The model under review builds one solid part; all positions refer to its coordinate system, in mm. Face numbers are marked on the shaded views. A direction names the side the tool comes from. Round coordinates to 2 decimals unless told otherwise and drop trailing zeros. Order: outer loops, then holes, each group sorted by start corner. A loop starts at its lowest first (then second) coordinate and runs counter-clockwise, first axis right, second up. Notation, with made-up numbers: M 8,24 L 39,24 A14 cw 39,31 Z; hole C 82.5,66 d7. An arc over 180 degrees is marked long. Use a Markdown table: item, result. Add a question column.
1. Insertion check: P1, Ø6, axis at x = 2.5, z = -22.5, coming from the +Y side; P2, Ø1, axis at x = -2, y = -2, coming from the -Z side; P3, Ø2, axis at x = 1, y = -0.5, coming from the -Z side; P4, Ø5.5, axis at x = 0.5, z = 0, coming from the -Y side. Each pin has a flat end and moves straight along its axis. Give the tip position at first contact, or say it passes through.
2. Consider section C-C on y = 0.75. State the section outline as (x, z) points.
3. Consider section A-A on x = 0. Count the separate pieces of the cut face and the enclosed holes in it, then the cut area to 3 significant figures.
4. Consider section B-B on z = 0. State the section outline as (x, y) points, then the cut area to 3 significant figures.
5. To check wall thickness, follow probe 1 along Z at (x, y) = (0, 0.15); probe 2 along Z at (x, y) = (0, -2); probe 3 along Y at (x, z) = (-2, -15.5). State the ranges of each line that lie inside material, in increasing order.
6. Consider section D-D on z = -21.5. State the section outline as (x, y) points, then the cut area to 3 significant figures.
7. For the marked faces 1, 2, 3, 4 and 5, list the 3-axis set-ups (+Z, -Z, +X, -X, +Y, -Y) from which the entire face can be reached by the end or side of a thin tool; tool diameter is ignored.
Autodesk Inventor part; units mm, degrees
ref_plane "Work Plane1" through (0, 1, 0) normal (0, -1, 0) x (1, 0, 0)
ref_plane "YZ Plane" through (0, 0, 0) normal (1, 0, 0) x (0, 1, 0)
ref_plane "XZ Plane" through (0, 0, 0) normal (0, 1, 0) x (-1, 0, 0)
sketch "Sketch1" plane through (0, 0, 0) normal (0, 1, 0) x (-1, 0, 0)
  arc A0 (6.9232, -1.0341) -> (-6.9232, -1.0341) centre (0, 0) ccw
  arc A1 (-3.7089, -22.554) -> (3.7089, -22.554) centre (0, -22) ccw
  line L0 (6.9232, -1.0341) -> (3.7089, -22.554)
  line L1 (-6.9232, -1.0341) -> (-3.7089, -22.554)
  circle A2 centre (0, -21.5) radius 0.5
  dimension "d0" = 14
  dimension "d1" = 7.5
  dimension "d2" = 22
  dimension "d3" = 1
  dimension "d4" = 21.5
extrude "Extrusion1" add sketch "Sketch1" along normal blind 2
sketch "Sketch2" plane through (0, 2, 0) normal (0, 1, 0) x (1, 0, 0)
  line L0 (-3.7089, 22.554) -> (-6.9232, 1.0341)
  line L1 (-5.8827, 8) -> (5.8827, 8)
  line L2 (6.9232, 1.0341) -> (3.7089, 22.554)
  arc A0 (-6.9232, 1.0341) -> (6.9232, 1.0341) centre (0, 0) ccw
  dimension "d7" = 8
extrude "Extrusion2" add sketch "Sketch2" along normal blind 1
chamfer "Chamfer1" distance 1 angle 45 3 edges at (6.403, 3, -4.517) (0, 3, 7) (-6.403, 3, -4.517)
chamfer "Chamfer2" distance 1 angle 45 1 edges at (0, 3, -8)
ref_plane "Work Plane1" through (0, 1, 0) normal (0, -1, 0) x (1, 0, 0)
mirror "Mirror1" about plane through (0, 1, 0) normal (0, -1, 0)
sketch "Sketch3" plane through (0, -1, 0) normal (0, -1, 0) x (1, 0, 0)
  circle A0 centre (0, 0) radius 5
  circle A1 centre (0, 0) radius 2.5
  dimension "d17" = 10
  dimension "d18" = 5
extrude "Extrusion3" add sketch "Sketch3" along normal blind 2
sketch "Sketch4" plane through (0, 3, 0) normal (0, 1, 0) x (1, 0, 0)
  point P0 (0, 0)
  point P1 (0, 0)
hole "Hole1" at (0, 3, 0) direction (0, -1, 0) diameter 2.5 depth 6
properties part number "5P.00.18.01-IB-VTP-Servo-Horn"
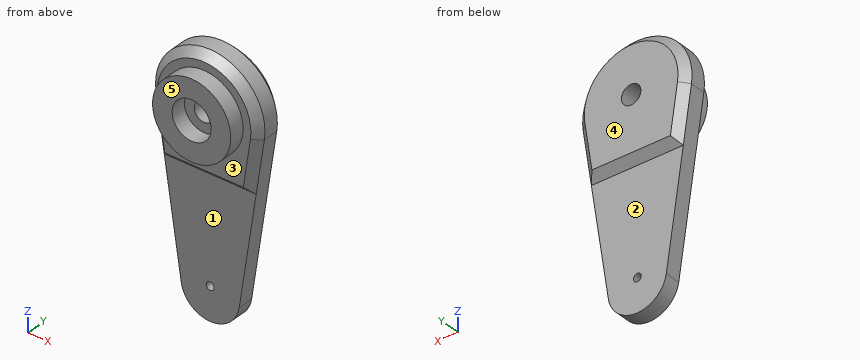
Answer block:
| question | item | result |
|---|---|---|
| 1 | P1 | y = 2 |
| 1 | P2 | z = -4.77 |
| 1 | P3 | z = -25.75 |
| 1 | P4 | y = -3 |
| 2 | outline | M -6.92,-1.03 L -3.71,-22.55 A3.75 ccw 3.71,-22.55 L 6.92,-1.03 A7 ccw long Z; hole C 0,0 d2.5; hole C 0,-21.5 d1 |
| 3 | separate pieces | 3 |
| 3 | enclosed holes | 0 |
| 3 | area | 91.5 mm^2 |
| 4 | outline | M -7,0 L -6,-1 L -5,-1 L -5,-3 L -2.5,-3 L -2.5,-1 L -1.25,-1 L -1.25,3 L -6,3 L -7,2 Z; M 1.25,-1 L 2.5,-1 L 2.5,-3 L 5,-3 L 5,-1 L 6,-1 L 7,0 L 7,2 L 6,3 L 1.25,3 Z |
| 4 | area | 54.0 mm^2 |
| 5 | probe 1 | -25.75 to -22, -21 to -1.25, 1.25 to 7 |
| 5 | probe 2 | -5 to -2.5, 2.5 to 5 |
| 5 | probe 3 | 0 to 2 |
| 6 | outline | M -3.87,0 L -0.5,0 L -0.5,2 L -3.87,2 Z; M 0.5,0 L 3.87,0 L 3.87,2 L 0.5,2 Z |
| 6 | area | 13.5 mm^2 |
| 7 | face 1 | -Z, +X, -X, -Y |
| 7 | face 2 | -Z, +X, -X, +Y |
| 7 | face 3 | -Y |
| 7 | face 4 | +Z, -Z, +X, -X, +Y |
| 7 | face 5 | +Z, -Z, +X, -X, -Y |
